Geometry check sheet. Reference: the model listing, model coordinates, mm. A direction names the side the tool comes from. Give positions to 0.01 mm unless a question says otherwise; leave off trailing zeros. Loops run counter-clockwise (first coordinate to the right, second up) from the corner with the lowest first, then second, coordinate; pieces in that order, holes last. Notation, with made-up numbers: (5.5, 52) - (38.5, 52) arc R19 ccw to (38.5, 85) - close; hole circle Ø10 at (-29.75, 71.5). An arc over 180 degrees is marked (long way). Use a Markdown table: item, result. Add a question column.
1. Depth check by flat-ended pin: P1, Ø10, axis at x = -4.5, y = 18, coming from the +Z side; P2, Ø5, axis at y = 24, z = 10, coming from the +X side; P3, Ø1.5, axis at y = 27, z = -13, coming from the -X side; P4, Ø10, axis at x = -11.5, y = 5.5, coming from the -Z side. Enter the tip coordinate at first touch or a pass-through.
2. Cross-section at B-B on y = 34. Enter the section's corners in (x, z) (1 decimal), and give its area (3 significant figures).
3. Set-up check for faces 1 (the cylindrical face through (-3.34, 39.62, 10.6)), 2 (the cylindrical face through (-1.38, 3.26, -6.2)), 3 (the flat face through (-11, 44.45, 3)): record each of +Z, -Z, +X, -X, +Y, -Y from which the full face is reachable in a straight line by a thin tool's end or side.
4. Material ranges on L1, parallel to X at y = 39, z = 0; L2, parallel to X at y = 40, z = 0; L3, parallel to Z at x = 0, y = 16.75, recorded low to high.
5. Draft check along Z on faces 4 (the conical face through (15.243, 44.053, 4.8)), 5 (the flat face through (0, 0, 0)), 6 (the conical face through (-0.807, 3.985, -0.179)). Enter one of: pulls with the +Z half, pulls with the -Z half, needs draft (parallel to the pull), parting line crosses it, or undercut.
6. Cross-section at A-A on y = 40. Enter the section's corners in (x, z) (1 decimal).
Autodesk Inventor part; units mm, degrees
ref_plane "YZ Plane" through (0, 0, 0) normal (1, 0, 0) x (0, 1, 0)
ref_plane "XZ Plane" through (0, 0, 0) normal (0, 1, 0) x (-1, 0, 0)
ref_plane "XY Plane" through (0, 0, 0) normal (0, 0, 1) x (1, 0, 0)
sketch "Sketch1" plane through (0, 0, 0) normal (0, 0, 1) x (1, 0, 0)
  line L0 (15.875, 44.45) -> (17.5765, 38.1)
  line L1 (17.5765, 38.1) -> (6.35, 6.35)
  line L2 (6.35, 6.35) -> (6.35, 0)
  line L3 (6.35, 0) -> (0, 0)
  line L4 (0, 0) -> (0, 44.45)
  line L5 (15.875, 44.45) -> (0, 44.45)
  dimension "d0" = 6.35
  dimension "d1" = 6.35
  dimension "d2" = 44.45
  dimension "d3" = 75
  dimension "d4" = 38.1
revolve "Revolution1" add sketch "Sketch1" angle 360 about axis through (0, 0, 0) along (0, 1, 0)
sketch "Sketch2" plane through (0, 44.45, 0) normal (0, 1, 0) x (1, 0, 0)
  point P0 (0, 0)
  point P1 (0, 0)
hole "Hole1" at (0, 44.45, 0) direction (0, -1, 0) diameter 9.525 depth 38.1 tip angle 118 counterbore diameter 22.225 counterbore depth 9.525
chamfer "Chamfer1" distance 0.254 angle 45 1 edges at (-6.35, 0, 0)
properties part number "Stack"
Values found:
| question | item | result |
|---|---|---|
| 1 | P1 | stops at z = 11.84 |
| 1 | P2 | stops at x = 10.41 |
| 1 | P3 | stops at x = -6.14 |
| 1 | P4 | passes through |
| 2 | outline | circle Ø32.3 at (0, 0); hole circle Ø9.5 at (0, 0) |
| 2 | area | 746 mm2 |
| 3 | face 1 | +Y |
| 3 | face 2 | -Y |
| 3 | face 3 | +Z, -Z, +X, -X, +Y |
| 4 | L1 | x = -17.34 to -11.11, 11.11 to 17.34 |
| 4 | L2 | x = -17.07 to -11.11, 11.11 to 17.07 |
| 4 | L3 | z = -10.03 to -4.76, 4.76 to 10.03 |
| 5 | face 4 | parting line crosses it |
| 5 | face 5 | needs draft |
| 5 | face 6 | undercut |
| 6 | outline | circle Ø34.1 at (0, 0); hole circle Ø22.2 at (0, 0) |
